Source: CAD feature listing. Evaluate the final solid. Frame: model axes, mm. Face numbers are marked on the shaded views. Coordinates: 2 decimals unless noted, no trailing zeros. Order: outer loops, then holes, each group sorted by start corner. A loop starts at its lowest first (then second) coordinate and runs counter-clockwise, first axis right, second up.
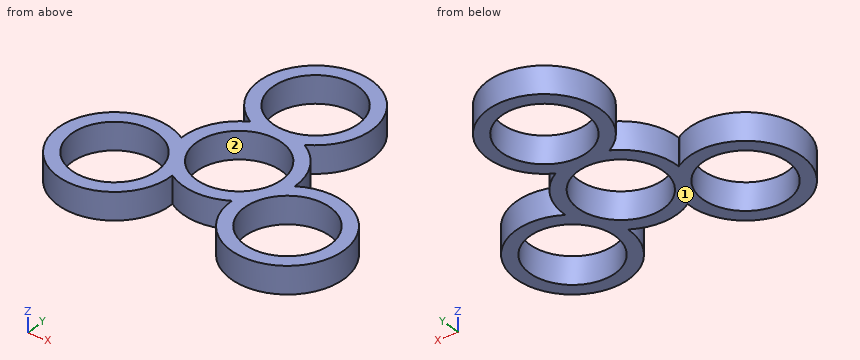
```python
from build123d import *

# Parameters (mm, degrees)
F1_R     = 10.9855
F2_DEPTH = 7


with BuildPart() as f2:
    # F1 (on Top) → F2 (new body)
    with BuildSketch(Plane.XY):
        with BuildLine():
            ThreePointArc((-14.480236, -0.390496), (-14.815783, -0.190689), (-15.156595, 0))
            ThreePointArc((-15.156595, 0), (-34.403537, -20.313797), (-7.578297, -12.345004))
            ThreePointArc((-7.578297, -12.345004), (0, -14.4855), (7.578297, -12.345004))
            ThreePointArc((7.578297, -12.345004), (34.603344, -19.97825), (14.480236, -0.390496))
            ThreePointArc((14.480236, -0.390496), (12.544811, 7.24275), (6.901938, 12.7355))
            ThreePointArc((6.901938, 12.7355), (0, 39.9565), (-6.901938, 12.7355))
            ThreePointArc((-6.901938, 12.7355), (-12.544811, 7.24275), (-14.480236, -0.390496))
        make_face()
        with Locations((-22.058533, -12.7355)):
            Circle(F1_R, mode=Mode.SUBTRACT)
        with Locations((22.058533, -12.7355)):
            Circle(F1_R, mode=Mode.SUBTRACT)
        Circle(F1_R, mode=Mode.SUBTRACT)
        with Locations((0, 25.471)):
            Circle(F1_R, mode=Mode.SUBTRACT)
    extrude(amount=F2_DEPTH)


solid = f2.part
```
1. Section query C-C on z = 5. Return loops of the section in (x, y) (1 decimal).
Findings:
outline: (-15.2, 0) arc R14.5 ccw (long way) to (-7.6, -12.3) arc R14.5 ccw to (7.6, -12.3) arc R14.5 ccw (long way) to (14.5, -0.4) arc R14.5 ccw to (6.9, 12.7) arc R14.5 ccw (long way) to (-6.9, 12.7) arc R14.5 ccw to (-14.5, -0.4) arc R14.5 ccw to start; hole circle Ø22 at (-22.1, -12.7); hole circle Ø22 at (0, 0); hole circle Ø22 at (0, 25.5); hole circle Ø22 at (22.1, -12.7)
2. Ray query, line 1 (Y direction, x = 0, z = 3.75); line 2 (X direction, y = -9, z = 6.25); line 3 (X direction, y = -8, z = 2.75). Return the intervals inside material, ascending.
Findings:
line 1: y = -14.49 to -10.99, 10.99 to 14.49, 36.46 to 39.96
line 2: x = -36.05 to -32.39, -11.73 to -6.3, 6.3 to 11.73, 32.39 to 36.05
line 3: x = -35.75 to -31.97, -12.15 to -7.53, 7.53 to 12.15, 31.97 to 35.75
3. Section query A-A on x = 0. Return loops of the section in (y, z), plus the area to 3 significant figures.
Findings:
outline: (-14.49, 0) - (-10.99, 0) - (-10.99, 7) - (-14.49, 7) - close; (10.99, 0) - (14.49, 0) - (14.49, 7) - (10.99, 7) - close; (36.46, 0) - (39.96, 0) - (39.96, 7) - (36.46, 7) - close
area: 73.5 mm2
4. Draft query along Y for the marked faces 1 and 2. Return one class per face: released by +Y, released by -Y, zero draft, split by the parting line, or undercut.
Findings:
face 1: zero draft
face 2: undercut
5. Section query D-D on y = 6. Return loops of the section in (x, z), plus the area to 3 significant figures.
Findings:
outline: (-13.18, 0) - (-9.2, 0) - (-9.2, 7) - (-13.18, 7) - close; (9.2, 0) - (13.18, 0) - (13.18, 7) - (9.2, 7) - close
area: 55.8 mm2
6. Section query B-B on y = -9. Return loops of the section in (x, z), plus the area to 3 significant figures.
Findings:
outline: (-36.05, 0) - (-32.39, 0) - (-32.39, 7) - (-36.05, 7) - close; (-11.73, 0) - (-6.3, 0) - (-6.3, 7) - (-11.73, 7) - close; (6.3, 0) - (11.73, 0) - (11.73, 7) - (6.3, 7) - close; (32.39, 0) - (36.05, 0) - (36.05, 7) - (32.39, 7) - close
area: 127 mm2
7. Pin query (flat end, axial travel): P1, Ø4, axis at y = 19, z = 2, coming from the +X side; P2, Ø1.5, axis at y = -11, z = 6, coming from the -X side. Return the tip coordinate at first contact, or that it passes through.
Findings:
P1: stops at x = 13.78
P2: stops at x = -36.51
